```python
from build123d import *

# Parameters (mm, degrees)
AUFSATZ_LINEAR_AUSTRAGEN1_DEPTH = 480
SKIZZE2_R                       = 2.75
SCHNITT_LINEAR_AUSTRAGEN1_DEPTH = 100
SKIZZE3_R                       = 2.75
SCHNITT_LINEAR_AUSTRAGEN2_DEPTH = 100
SKIZZE4_R                       = 2.75
SCHNITT_LINEAR_AUSTRAGEN3_DEPTH = 10
SKIZZE5_R                       = 2.5
SCHNITT_LINEAR_AUSTRAGEN4_DEPTH = 60
SKIZZE6_R                       = 2.5
SCHNITT_LINEAR_AUSTRAGEN5_DEPTH = 100


with BuildPart() as part:
    # Skizze1 → Aufsatz-Linear austragen1 (new, symmetric)
    with BuildSketch(Plane.XY):
        with BuildLine():
            Line((-14, 20), (14, 20))
            ThreePointArc((14, 20), (18.242640687, 18.242640687), (20, 14))
            Line((20, 14), (20, -14))
            ThreePointArc((20, -14), (18.242640687, -18.242640687), (14, -20))
            Line((14, -20), (-14, -20))
            ThreePointArc((-14, -20), (-18.242640687, -18.242640687), (-20, -14))
            Line((-20, -14), (-20, 14))
            ThreePointArc((-20, 14), (-18.242640687, 18.242640687), (-14, 20))
        make_face()
        with BuildLine():
            Line((-18, 14), (-18, -14))
            ThreePointArc((-18, -14), (-16.828427125, -16.828427125), (-14, -18))
            Line((-14, -18), (14, -18))
            ThreePointArc((14, -18), (16.828427125, -16.828427125), (18, -14))
            Line((18, -14), (18, 14))
            ThreePointArc((18, 14), (16.828427125, 16.828427125), (14, 18))
            Line((14, 18), (-14, 18))
            ThreePointArc((-14, 18), (-16.828427125, 16.828427125), (-18, 14))
        make_face(mode=Mode.SUBTRACT)
    extrude(amount=AUFSATZ_LINEAR_AUSTRAGEN1_DEPTH, both=True)

    # Skizze2 → Schnitt-Linear austragen1 (cut)
    with BuildSketch(Plane(origin=(0, 20, 0), x_dir=(1, 0, 0), z_dir=(0, 1, 0))):
        with Locations(Location((0, 460, 0), (0, 0, 270))):
            Circle(SKIZZE2_R)
        with Locations((0, -460)):
            Circle(SKIZZE2_R)
    extrude(amount=-SCHNITT_LINEAR_AUSTRAGEN1_DEPTH, mode=Mode.SUBTRACT)

    # Skizze3 → Schnitt-Linear austragen2 (cut)
    with BuildSketch(Plane(origin=(20, 0, 0), x_dir=(0, 0, -1), z_dir=(1, 0, 0))):
        with Locations((460, 0)):
            Circle(SKIZZE3_R)
        with Locations(Location((-460, 0, 0), (0, 0, 180))):
            Circle(SKIZZE3_R)
    extrude(amount=-SCHNITT_LINEAR_AUSTRAGEN2_DEPTH, mode=Mode.SUBTRACT)

    # Skizze4 → Schnitt-Linear austragen3 (cut)
    with BuildSketch(Plane(origin=(20, 0, 0), x_dir=(0, 0, -1), z_dir=(1, 0, 0))):
        with Locations((409, -2.5)):
            Circle(SKIZZE4_R)
        with Locations((394, -2.5)):
            Circle(SKIZZE4_R)
        with Locations((-348, -2.5)):
            Circle(SKIZZE4_R)
    extrude(amount=-SCHNITT_LINEAR_AUSTRAGEN3_DEPTH, mode=Mode.SUBTRACT)

    # Skizze5 → Schnitt-Linear austragen4 (cut)
    with BuildSketch(Plane(origin=(0, 20, 0), x_dir=(1, 0, 0), z_dir=(0, 1, 0))):
        with Locations(Location((0, 270, 0), (0, 0, 270))):
            Circle(SKIZZE5_R)
        with Locations(Location((0, 90, 0), (0, 0, 270))):
            Circle(SKIZZE5_R)
        with Locations((0, -270)):
            Circle(SKIZZE5_R)
        with Locations((0, -90)):
            Circle(SKIZZE5_R)
    extrude(amount=-SCHNITT_LINEAR_AUSTRAGEN4_DEPTH, mode=Mode.SUBTRACT)

    # Skizze6 → Schnitt-Linear austragen5 (cut)
    with BuildSketch(Plane.ZY.offset(20)):
        with Locations((270, 0)):
            Circle(SKIZZE6_R)
        with Locations((90, 0)):
            Circle(SKIZZE6_R)
        with Locations((-270, 0)):
            Circle(SKIZZE6_R)
        with Locations((-90, 0)):
            Circle(SKIZZE6_R)
    extrude(amount=-SCHNITT_LINEAR_AUSTRAGEN5_DEPTH, mode=Mode.SUBTRACT)


solid = part.part
```
Geometry check sheet. Reference: the model listing, model coordinates, mm. A direction names the side the tool comes from. Round coordinates to 2 decimals unless told otherwise and drop trailing zeros. Loops run counter-clockwise (first coordinate to the right, second up) from the corner with the lowest first, then second, coordinate; pieces in that order, holes last. Notation, with made-up numbers: (-33, -24.5) -> (19, -24.5) arc R14 cw to (19, -2.5) -> close; hole circle Ø3 at (55, 9.25). An arc over 180 degrees is marked (long way). Use a Markdown table: item, result.
(1) Scan lines: probe 1 along Y at (x, z) = (-3, -22.5); probe 2 along X at (y, z) = (-18.55, 270). Record each from-to range of solid material in increasing order.
Calculated:
| item | result |
|---|---|
| probe 1 | -20 to -18, 18 to 20 |
| probe 2 | -17.91 to -2.5, 2.5 to 17.91 |
(2) Sectioned sample at A-A (z = 164). Enter the section's corners in (x, y).
Calculated:
| item | result |
|---|---|
| outline | (-20, -14) arc R6 ccw to (-14, -20) -> (14, -20) arc R6 ccw to (20, -14) -> (20, 14) arc R6 ccw to (14, 20) -> (-14, 20) arc R6 ccw to (-20, 14) -> close; hole (-18, -14) arc R4 ccw to (-14, -18) -> (14, -18) arc R4 ccw to (18, -14) -> (18, 14) arc R4 ccw to (14, 18) -> (-14, 18) arc R4 ccw to (-18, 14) -> close |
(3) Mould release check, pull along Y, two halves, no side actions. Record for faces 1 (the flat face through (0, 20, 7)), 2 (the flat face through (2, -19, -480)), 3 (the flat face through (18, 0, 7)), 4 (the flat face through (0, 18, 7)): released by +Y, released by -Y, zero draft, split by the parting line, or undercut.
Calculated:
| item | result |
|---|---|
| face 1 | released by +Y |
| face 2 | zero draft |
| face 3 | undercut |
| face 4 | undercut |
(4) Set-up check for faces 5 (the flat face through (-18, 0, 7)), 6 (the flat face through (-20, 0, 7)): record each of +Z, -Z, +X, -X, +Y, -Y from which the full face is reachable in a straight line by a thin tool's end or side.
Calculated:
| item | result |
|---|---|
| face 5 | +Z, -Z |
| face 6 | +Z, -Z, -X, +Y, -Y |
